Can you work these out from the model? Positions are in its coordinate system, mm. Face numbers are marked on the shaded views. A direction names the side the tool comes from. Coordinates: 2 decimals unless noted, no trailing zeros. Loops run counter-clockwise (first coordinate to the right, second up) from the corner with the lowest first, then second, coordinate; pieces in that order, holes last. Notation, with made-up numbers: M 18.5,-9.5 L 45.5,-9.5 A23 ccw 45.5,21.5 Z; hole C 17,-25 d5. An arc over 180 degrees is marked long. Answer as a JSON object with one key per item and string values. Group by question number.
Item 1: Suppose I cut it at A-A (z = -0.35). Write out the boundary of the cut face in (x, y), then the cut area to 3 significant figures.
Item 2: We'd pull the mould along Z, two halves only. Please class the marked faces 1, 2 and 3: +Z half, -Z half, draft (parallel to the pull), parting line (faces both ways), or undercut.
Item 3: Which directions (+Z, -Z, +X, -X, +Y, -Y) give clear straight access to the entire face, cutting with the end or side of a thin tool? Please do the marked faces 4 and 5.
Item 4: Suppose I cut it at D-D (x = 26.5). Write out the boundary of the cut face in (y, z), then the cut area to 4 significant figures.
Item 5: If I drill on line 1 (X direction, y = 3.75, z = -1.8); line 2 (X direction, y = 11.5, z = -2.05); line 3 (Z direction, x = 30.5, y = 9.5), over which ranges is the centre line in solid material (lowest first)?
Item 6: I'm going to push a flat-ended pin straight in: pin 1 Ø3.5 at (x, z) = (26.5, -2.5) entering from +Y. Where does the tip first touch, or does it pass through?
Item 7: Suppose I cut it at C-C (y = 4.75). Write out the boundary of the cut face in (x, z), then the cut area to 3 significant figures.
Item 8: Suppose I cut it at B-B (x = 21). Write out the boundary of the cut face in (y, z), then the cut area to 4 significant figures.
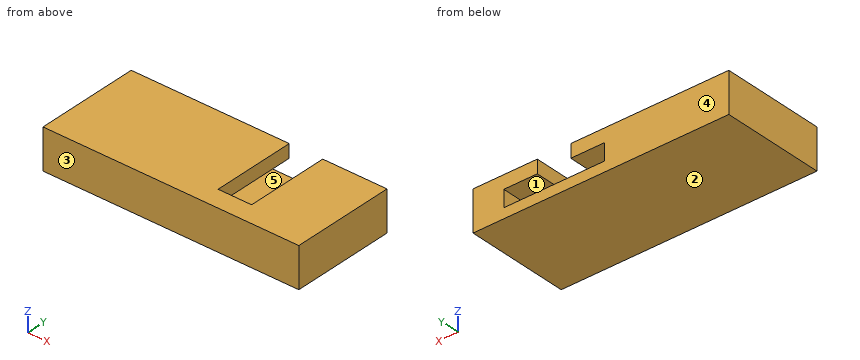
```python
from build123d import *

# Parameters (mm, degrees)
SKETCH2_W           = 39
SKETCH2_H           = 15.5
BOSS_EXTRUDE1_DEPTH = 6
CUT_EXTRUDE1_DEPTH  = 12.5
SKETCH4_W           = 20.319843286
SKETCH4_H           = 28.236665345
CUT_EXTRUDE2_DEPTH  = 0.4
SKETCH5_W           = 11.083550883
SKETCH5_H           = 22.584934042
CUT_EXTRUDE3_DEPTH  = 0.4


with BuildPart() as part:
    # Sketch2 → Boss-Extrude1 (new body)
    with BuildSketch(Plane.XY):
        with Locations((19.5, 7.75)):
            Rectangle(SKETCH2_W, SKETCH2_H)
    extrude(amount=-BOSS_EXTRUDE1_DEPTH)

    # Sketch3 → Cut-Extrude1 (cut)
    with BuildSketch(Plane(origin=(0, 15.5, 0), x_dir=(1, 0, 0), z_dir=(0, 1, 0))):
        Polygon((24, 0), (24, 2), (19, 2), (19, 4.5), (34, 4.5), (34, 2), (29, 2), (29, 0), align=None)
    extrude(amount=-CUT_EXTRUDE1_DEPTH, mode=Mode.SUBTRACT)

    # Sketch4 → Cut-Extrude2 (cut)
    with BuildSketch(Plane(origin=(39, 0, 0), x_dir=(0, 0, -1), z_dir=(1, 0, 0))):
        with Locations((6.654932851, 5.177032831)):
            Rectangle(SKETCH4_W, SKETCH4_H)
    extrude(amount=-CUT_EXTRUDE2_DEPTH, mode=Mode.SUBTRACT)

    # Sketch5 → Cut-Extrude3 (cut)
    with BuildSketch(Plane.ZY):
        with Locations((-2.571172138, 7.134247173)):
            Rectangle(SKETCH5_W, SKETCH5_H)
    extrude(amount=-CUT_EXTRUDE3_DEPTH, mode=Mode.SUBTRACT)


solid = part.part
```
From the geometry:
{
 "1": {"outline": "M 0.4,0 L 38.6,0 L 38.6,15.5 L 29,15.5 L 29,3 L 24,3 L 24,15.5 L 0.4,15.5 Z", "area": "530 mm2"},
 "2": {"face 1": "undercut", "face 2": "-Z half", "face 3": "draft"},
 "3": {"face 4": "+Z, -Z, +X, -X, +Y", "face 5": "+Y"},
 "4": {"outline": "M 0,-6 L 15.5,-6 L 15.5,-4.5 L 3,-4.5 L 3,0 L 0,0 Z", "area": "36.75 mm2"},
 "5": {"line 1": "0.4 to 24, 29 to 38.6", "line 2": "0.4 to 19, 34 to 38.6", "line 3": "-6 to -4.5, -2 to 0"},
 "6": {"pin 1": "y = 3"},
 "7": {"outline": "M 0.4,-6 L 38.6,-6 L 38.6,0 L 29,0 L 29,-2 L 34,-2 L 34,-4.5 L 19,-4.5 L 19,-2 L 24,-2 L 24,0 L 0.4,0 Z", "area": "182 mm2"},
 "8": {"outline": "M 0,-6 L 15.5,-6 L 15.5,-4.5 L 3,-4.5 L 3,-2 L 15.5,-2 L 15.5,0 L 0,0 Z", "area": "61.75 mm2"}
}
